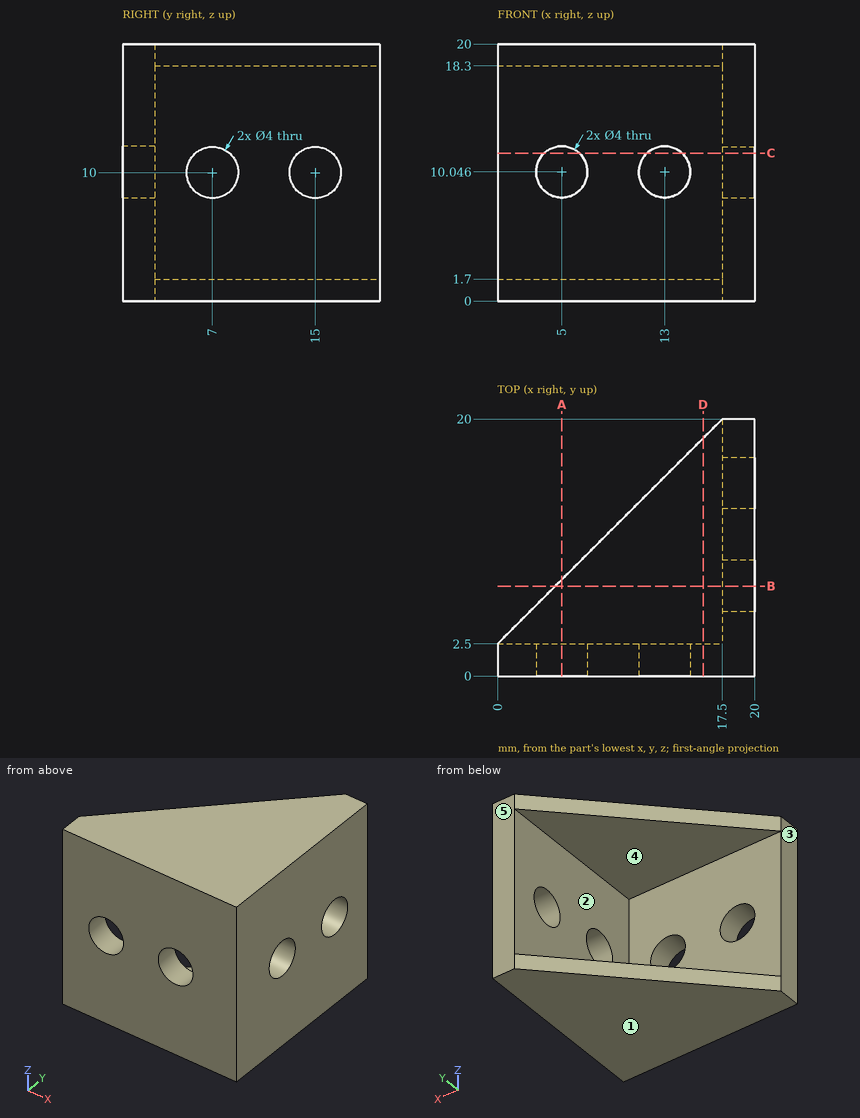
Here's the drawing with two shaded views (mm, measured from the low corner). I have some questions. A direction names the side the tool comes from. Give positions to 0.01 mm unless a question says otherwise; leave off trailing zeros. Loops run counter-clockwise (first coordinate to the right, second up) from the corner with the lowest first, then second, coordinate; pieces in that order, holes last. Notation, with made-up numbers: M 73.25,43 L 90.25,43 A19 cw 90.25,52 Z; hole C 66.25,5 d7. An arc over 180 degrees is marked long. Use one line per item in the form item = value. Start each with the question number.
Q1. If we section it at D-D (x = 16): Write out the boundary of the cut face in (y, z), then the cut area to 3 significant figures.
Q2. Thinking about a two-plate mould opening in Z: for the marked faces 1, 2 and 3, which applies, +Z half, -Z half, draft (parallel to the pull), parting line (faces both ways), or undercut?
Q3. Will these pins go through, and if not, where does the flat tip stop? pin 1 Ø1.5 at (x, z) = (13.5, 15) entering from +Y; pin 2 Ø5 at (y, z) = (13.5, 3.5) entering from -X (3 decimals); pin 3 Ø1.5 at (y, z) = (15.5, 10) entering from -X; pin 4 Ø4.5 at (y, z) = (15, 10) entering from -X.
Q4. Which directions (+Z, -Z, +X, -X, +Y, -Y) give clear straight access to the entire face, cutting with the end or side of a thin tool? Please do the marked faces 4 and 5.
Q5. If we section it at B-B (y = 7): Write out the boundary of the cut face in (x, z), then the cut area to 3 significant figures.
Q6. If we section it at C-C (z = 11.5): Write out the boundary of the cut face in (x, y), then the cut area to 3 significant figures.
Q7. I need wall thicknesses on line 1 along Y through (x, z) = (18.6, 10); line 2 along Z through (x, y) = (13, 3); line 3 along X through (y, z) = (18.25, 9.25). Which ranges of each line are inside material? Lowest first, please.
Q8. If we section it at A-A (x = 5): Write out the boundary of the cut face in (y, z), then the cut area to 3 significant figures.
Taken from the geometry:
q1.outline = M 0,0 L 18.5,0 L 18.5,1.7 L 2.5,1.7 L 2.5,18.3 L 18.5,18.3 L 18.5,20 L 0,20 Z
q1.area = 104 mm^2
q2.face_1 = -Z half
q2.face_2 = undercut
q2.face_3 = draft
q3.pin_1 = 2.5
q3.pin_2 = 9.265
q3.pin_3 = through
q3.pin_4 = 17.5
q4.face_4 = -X, +Y
q4.face_5 = +Z, -Z, +X, -X, +Y
q5.outline = M 4.5,0 L 20,0 L 20,8 L 17.5,8 L 17.5,1.7 L 4.5,1.7 Z; M 4.5,18.3 L 17.5,18.3 L 17.5,12 L 20,12 L 20,20 L 4.5,20 Z
q5.area = 84.2 mm^2
q6.outline = M 0,0 L 3.63,0 L 3.63,2.5 L 0,2.5 Z; M 6.37,0 L 11.63,0 L 11.63,2.5 L 6.37,2.5 Z; M 14.37,0 L 20,0 L 20,5.68 L 17.5,5.68 L 17.5,2.5 L 14.37,2.5 Z; M 17.5,8.32 L 20,8.32 L 20,13.68 L 17.5,13.68 Z; M 17.5,16.32 L 20,16.32 L 20,20 L 17.5,20 Z
q6.area = 66.8 mm^2
q7.line_1 = 0 to 5, 9 to 13, 17 to 20
q7.line_2 = 0 to 1.7, 18.3 to 20
q7.line_3 = 17.5 to 20
q8.outline = M 0,0 L 7.5,0 L 7.5,1.7 L 2.5,1.7 L 2.5,8.05 L 0,8.05 Z; M 0,12.05 L 2.5,12.05 L 2.5,18.3 L 7.5,18.3 L 7.5,20 L 0,20 Z
q8.area = 57.0 mm^2
